Part model, mm, in its own coordinate system. Face numbers are marked on the shaded views. A direction names the side the tool comes from. Give positions to 0.01 mm unless a question says otherwise; leave off trailing zeros. Order: outer loops, then holes, each group sorted by start corner. A loop starts at its lowest first (then second) coordinate and runs counter-clockwise, first axis right, second up.
from build123d import *

# Parameters (mm, degrees)
BOSS_EXTRUDE1_DEPTH = 5.842
CUT_EXTRUDE1_DEPTH  = 36.478423215


with BuildPart() as part:
    # Sketch1 → Boss-Extrude1 (new body)
    with BuildSketch(Plane.XY):
        Polygon((21.1058, -20.928), (21.1058, -19.15), (26.9478, -19.15), (26.9478, -6.25), (21.1058, -6.25), (21.1058, -1.778), (14.7558, -1.778), (14.7558, -3.96875), (11.977675, -3.96875), (11.977675, -1.778), (7.8978, -1.778), (7.8978, 1.778), (11.977675, 1.778), (11.977675, 3.96875), (14.7558, 3.96875), (14.7558, 1.778), (21.1058, 1.778), (21.1058, 6.25), (26.9478, 6.25), (26.9478, 19.15), (21.1058, 19.15), (21.1058, 22.325), (-21.1058, 22.325), (-21.1058, 19.15), (-26.9478, 19.15), (-26.9478, 6.25), (-21.1058, 6.25), (-21.1058, 1.778), (-14.7558, 1.778), (-14.7558, 3.96875), (-11.977675, 3.96875), (-11.977675, 1.778), (-7.8978, 1.778), (-7.8978, -1.778), (-11.977675, -1.778), (-11.977675, -3.96875), (-14.7558, -3.96875), (-14.7558, -1.778), (-21.1058, -1.778), (-21.1058, -6.25), (-26.9478, -6.25), (-26.9478, -19.15), (-21.1058, -19.15), (-21.1058, -20.928), align=None)
    extrude(amount=BOSS_EXTRUDE1_DEPTH)

    # Sketch2 → Cut-Extrude1 (cut, through all)
    with BuildSketch(Plane.XY.offset(5.842)):
        with BuildLine():
            Line((-9.525, 17.4625), (9.525, 17.4625))
            ThreePointArc((9.525, 17.4625), (14.2875, 12.7), (9.525, 7.9375))
            Line((9.525, 7.9375), (-9.525, 7.9375))
            ThreePointArc((-9.525, 7.9375), (-14.2875, 12.7), (-9.525, 17.4625))
        make_face()
        with BuildLine():
            Line((-9.525, -17.4625), (9.525, -17.4625))
            ThreePointArc((9.525, -17.4625), (14.2875, -12.7), (9.525, -7.9375))
            Line((9.525, -7.9375), (-9.525, -7.9375))
            ThreePointArc((-9.525, -7.9375), (-14.2875, -12.7), (-9.525, -17.4625))
        make_face()
    extrude(amount=-CUT_EXTRUDE1_DEPTH, mode=Mode.SUBTRACT)


solid = part.part
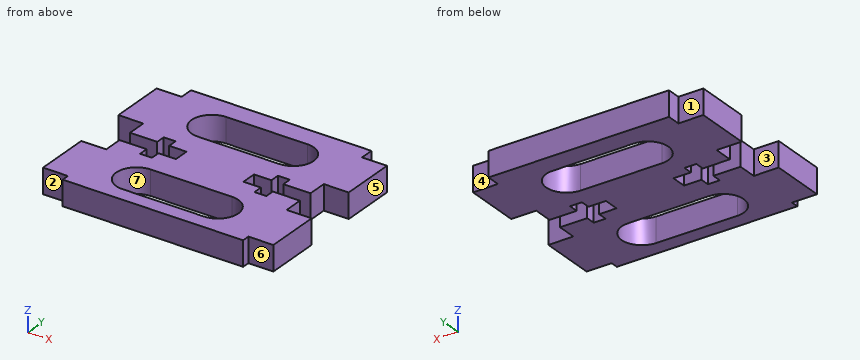
Item 1: Band-saw the part on A-A on y = 12.7. List the corners of the cut face in (x, z).
Item 2: Band-saw the part on B-B on x = -22. List the corners of the cut face in (y, z), plus the area to 3 significant figures.
Item 3: Band-saw the part on D-D on z = 4.6. Give the number of separate pieces and of enclosed holes in the cut face, plus the area to 3 significant figures.
Item 4: Drop flat-ended pins along their axis: P1, Ø1.8, axis at x = 23, z = 2.5, coming from the -Y side; P2, Ø2, axis at y = 0.5, z = 3.5, coming from the -X side; P3, Ø0.7, axis at y = 3.5, z = 2.5, coming from the +X side. Give the stop position or say it passes through.
Item 5: Which spindle directions (+Z, -Z, +X, -X, +Y, -Y) get a long thin tool onto all of the face, cutting with end or side? Do the marked faces 1, 2, 3 and 4. Say none if no direction does.
Item 6: Band-saw the part on C-C on x = 3. List the corners of the cut face in (y, z) (1 decimal).
Item 7: Drill centre lines: probe 1 along Y at (x, z) = (-3.5, 0.65) (1 decimal); probe 2 along X at (y, z) = (-2, 0.8); probe 3 along Y at (x, z) = (18, 0.5) (3 decimals). Where is each one in solid material? Low to high.
Item 8: Pull direction X, two halves, no side cores. Call the marked faces 5, 6 and 7: released by +X, released by -X, zero draft, split by the parting line, or undercut.
Working result:
1. outline: (-26.95, 0) - (-14.29, 0) - (-14.29, 5.84) - (-26.95, 5.84) - close; (14.29, 0) - (26.95, 0) - (26.95, 5.84) - (14.29, 5.84) - close
2. outline: (-19.15, 0) - (-6.25, 0) - (-6.25, 5.84) - (-19.15, 5.84) - close; (6.25, 0) - (19.15, 0) - (19.15, 5.84) - (6.25, 5.84) - close
2. area: 151 mm2
3. separate pieces: 1
3. enclosed holes: 2
3. area: 1,500 mm2
4. P1: stops at y = -19.15
4. P2: stops at x = -7.9
4. P3: stops at x = 21.11
5. face 1: +Z, -Z, -X, +Y
5. face 2: +Z, -Z, -X, -Y
5. face 3: +Z, -Z, -X
5. face 4: +Z, -Z, +X, +Y
6. outline: (-20.9, 0) - (-17.5, 0) - (-17.5, 5.8) - (-20.9, 5.8) - close; (-7.9, 0) - (7.9, 0) - (7.9, 5.8) - (-7.9, 5.8) - close; (17.5, 0) - (22.3, 0) - (22.3, 5.8) - (17.5, 5.8) - close
7. probe 1: y = -20.9 to -17.5, -7.9 to 7.9, 17.5 to 22.3
7. probe 2: x = -21.11 to -14.76, -11.98 to 11.98, 14.76 to 21.11
7. probe 3: y = -20.928 to -1.778, 1.778 to 22.325
8. face 5: released by +X
8. face 6: zero draft
8. face 7: undercut
